The model under review builds one solid part; all positions refer to its coordinate system, in mm. A direction names the side the tool comes from. Round coordinates to 2 decimals unless told otherwise and drop trailing zeros. Loops run counter-clockwise (first coordinate to the right, second up) from the corner with the lowest first, then second, coordinate; pieces in that order, holes last. Notation, with made-up numbers: M -9.5,14.25 L 28.5,14.25 A21 ccw 28.5,28.25 Z; hole C -39,42 d1. An arc over 180 degrees is marked long. One line per question, with ' | ' between items.
from build123d import *

# Parameters (mm, degrees)
SKETCH1_W                    = 50.8
SKETCH1_H                    = 50.8
EXTRUDE1_DEPTH               = 38.1
SKETCH2_R                    = 12.7
EXTRUDE2_DEPTH               = 69.391593051
F_1_2_CLEARANCE_HOLE1_D      = 13.89126
F_1_4_20_TAPPED_HOLE1_REACH  = 92.482
F_1_4_20_TAPPED_HOLE1_BORE_R = 2.5527


with BuildPart() as part:
    # Sketch1 → Extrude1 (new, symmetric)
    with BuildSketch(Plane.XY):
        Rectangle(SKETCH1_W, SKETCH1_H)
    extrude(amount=EXTRUDE1_DEPTH, both=True)

    # Sketch2 → Extrude2 (cut, through all)
    with BuildSketch(Plane(origin=(25.4, 0, 0), x_dir=(0, 0, -1), z_dir=(1, 0, 0))):
        with Locations((0, 5.08)):
            Circle(SKETCH2_R)
    extrude(amount=-EXTRUDE2_DEPTH, mode=Mode.SUBTRACT)

    # 1/2 Clearance Hole1 (through all)
    with Locations(Plane(origin=(0, 25.4, 21.59), x_dir=(0, 0, 1), z_dir=(0, 1, 0))):
        with Locations((0, 0)):
            f_1_2_clearance_hole1 = Hole(F_1_2_CLEARANCE_HOLE1_D / 2)

    # Mirror1: 1/2 Clearance Hole1 across plane
    add(f_1_2_clearance_hole1.mirror(Plane.XY), mode=Mode.SUBTRACT)

    # 1/4-20 Tapped Hole1 bore (on position points) → 1/4-20 Tapped Hole1 (cut, up to next)
    with BuildSketch(Plane(origin=(12.7, 5.08, -38.1), x_dir=(-1, 0, 0), z_dir=(0, 0, -1)), mode=Mode.PRIVATE) as f_1_4_20_tapped_hole1_sk1:
        Circle(F_1_4_20_TAPPED_HOLE1_BORE_R)
    f_1_4_20_tapped_hole1_tool1 = extrude(f_1_4_20_tapped_hole1_sk1.sketch, amount=-F_1_4_20_TAPPED_HOLE1_REACH, mode=Mode.PRIVATE) & part.part
    f_1_4_20_tapped_hole1 = f_1_4_20_tapped_hole1_tool1.solids().sort_by_distance((12.7, 5.08, -38.1))[0]
    add(f_1_4_20_tapped_hole1, mode=Mode.SUBTRACT)

    # Mirror2: 1/4-20 Tapped Hole1 across plane
    add(f_1_4_20_tapped_hole1.mirror(Plane(origin=(0, 0, 0), x_dir=(0, 0, 1), z_dir=(1, 0, 0))), mode=Mode.SUBTRACT)


solid = part.part
1) Mouldability with a two-part tool opening along X and no side actions: class faces 3 (the flat face through (25.4, -6, 9)), 4 (the cylindrical face through (2.086, -0.356, 14.965)), 5 (the flat face through (0, -25.4, 1)) as +X half, -X half, draft (parallel to the pull), parting line (faces both ways), or undercut.
Output values:
face 3: +X half | face 4: undercut | face 5: draft
2) For line 1 (Y direction, x = -12.7, z = -18.5); line 2 (X direction, y = -5, z = -21.59); line 3 (Z direction, x = -2, y = 16), list the stretches that pass through material, from the lowest coordinate up.
Output values:
line 1: y = -25.4 to 2.53, 7.63 to 25.4 | line 2: x = -25.4 to -6.95, 6.95 to 25.4 | line 3: z = -38.1 to -28.24, -14.94 to -6.48, 6.48 to 14.94, 28.24 to 38.1
3) Machinability: for faces 1 (the flat face through (0, 0, -38.1)), 2 (the cylindrical face through (-10.265, 5.847, -25.45)), which of the approach directions +Z, -Z, +X, -X, +Y, -Y give a long, thin tool a straight path to every point of the face, cutting with its end or side? Answer none if there is none.
Output values:
face 1: -Z, +X, -X, +Y, -Y | face 2: -Z
4) Add section C-C on z = 21.59. State the section outline as (x, y) points.
Output values:
outline: M -25.4,-25.4 L -6.95,-25.4 L -6.95,25.4 L -25.4,25.4 Z; M 6.95,-25.4 L 25.4,-25.4 L 25.4,25.4 L 6.95,25.4 Z
5) Add section A-A on x = 0. State the section outline as (y, z) points, then the cut area to 3 significant figures.
Output values:
outline: M -25.4,-38.1 L 25.4,-38.1 L 25.4,-28.54 L -25.4,-28.54 Z; M -25.4,-14.64 L 25.4,-14.64 L 25.4,14.64 L -25.4,14.64 Z; M -25.4,28.54 L 25.4,28.54 L 25.4,38.1 L -25.4,38.1 Z; hole C 5.08,0 d25.4 | area: 1,950 mm²
6) Add section D-D on y = 0. State the section outline as (x, z) points.
Output values:
outline: M -25.4,-38.1 L 25.4,-38.1 L 25.4,-11.64 L -25.4,-11.64 Z; M -25.4,11.64 L 25.4,11.64 L 25.4,38.1 L -25.4,38.1 Z; hole C 0,-21.59 d13.89; hole C 0,21.59 d13.89
7) Add section B-B on z = -21.59. State the section outline as (x, y) points.
Output values:
outline: M -25.4,-25.4 L -6.95,-25.4 L -6.95,25.4 L -25.4,25.4 Z; M 6.95,-25.4 L 25.4,-25.4 L 25.4,25.4 L 6.95,25.4 Z; hole C -12.7,5.08 d5.11; hole C 12.7,5.08 d5.11
